Design review of the part built by this model. Coordinates are the model's own, in mm. A direction names the side the tool comes from. Coordinates: 2 decimals unless noted, no trailing zeros. Loops run counter-clockwise (first coordinate to the right, second up) from the corner with the lowest first, then second, coordinate; pieces in that order, holes last. Notation, with made-up numbers: (87, -32) - (120, -32) arc R23 cw to (120, -22) - close; hole circle Ø4 at (59, 80.25). An arc over 180 degrees is marked (long way). Return JSON: item names as keys, results as strings. Group by question number.
from build123d import *

# Parameters (mm, degrees)
BOSS_EXTRUDE1_DEPTH = 5.588
CUT_EXTRUDE1_REACH  = 80.367
SKETCH2_W           = 75.3618
SKETCH2_H           = 1.524
SKETCH3_W           = 8.255
SKETCH3_H           = 10.8204
CUT_EXTRUDE2_DEPTH  = 83.86461998


with BuildPart() as part:
    # Sketch1 → Boss-Extrude1 (new, symmetric)
    with BuildSketch(Plane.XY):
        Polygon((37.6809, 28.1432), (-37.6809, 28.1432), (-37.6809, 34.109215507), (-52.6415, 34.109215507), (-52.6415, 21.028215507), (-29.263085056, 21.028215507), (-18.341239915, -12.742623419), (-18.341239915, -29.6418), (-10.721239915, -29.6418), (-2.406356809, -15.24), (2.406356809, -15.24), (10.721239915, -29.6418), (18.341239915, -29.6418), (18.341239915, -12.742623419), (29.263085056, 21.028215507), (52.6415, 21.028215507), (52.6415, 34.109215507), (37.6809, 34.109215507), align=None)
        with BuildLine():
            Line((11.480303153, -7.62), (-11.480303153, -7.62))
            ThreePointArc((-11.480303153, -7.62), (-13.362052491, -6.011722817), (-12.066505741, -3.902435097))
            Line((-12.066505741, -3.902435097), (0, 0))
            Line((0, 0), (12.066505741, -3.902435097))
            ThreePointArc((12.066505741, -3.902435097), (13.362052491, -6.011722817), (11.480303153, -7.62))
        make_face(mode=Mode.SUBTRACT)
        Polygon((20.32, 22.225), (-20.32, 22.225), (0, 7.62), align=None, mode=Mode.SUBTRACT)
        Polygon((-21.301071122, 15.641859193), (-5.650084624, 4.392712647), (-16.52547404, 0.87549712), align=None, mode=Mode.SUBTRACT)
        Polygon((16.52547404, 0.87549712), (21.301071122, 15.641859193), (5.650084624, 4.392712647), align=None, mode=Mode.SUBTRACT)
    extrude(amount=BOSS_EXTRUDE1_DEPTH, both=True)

    # Cut-Extrude1: up to this face of the body (flat: up to its plane)
    cut_extrude1_end = Plane(part.part.faces().sort_by_distance((-14.531239915, -29.6418, 0))[0])
    # Sketch2 → Cut-Extrude1 (cut, up to the picked face)
    with BuildSketch(Plane(origin=(0, 28.1432, 0), x_dir=(1, 0, 0), z_dir=(0, 1, 0)), mode=Mode.PRIVATE) as cut_extrude1_sk1:
        with Locations((0, -4.826)):
            Rectangle(SKETCH2_W, SKETCH2_H)
    cut_extrude1_tool1 = split(extrude(cut_extrude1_sk1.sketch, amount=-CUT_EXTRUDE1_REACH, mode=Mode.PRIVATE), bisect_by=cut_extrude1_end, keep=Keep.BOTH, mode=Mode.PRIVATE)
    # Sketch2 → Cut-Extrude1 (cut, up to the picked face)
    with BuildSketch(Plane(origin=(0, 28.1432, 0), x_dir=(1, 0, 0), z_dir=(0, 1, 0)), mode=Mode.PRIVATE) as cut_extrude1_sk2:
        with Locations((0, 4.826)):
            Rectangle(SKETCH2_W, SKETCH2_H)
    cut_extrude1_tool2 = split(extrude(cut_extrude1_sk2.sketch, amount=-CUT_EXTRUDE1_REACH, mode=Mode.PRIVATE), bisect_by=cut_extrude1_end, keep=Keep.BOTH, mode=Mode.PRIVATE)
    add(cut_extrude1_tool1.solids().sort_by(Axis((0, 28.1432, 4.826), (0, -1, 0)))[0], mode=Mode.SUBTRACT)
    add(cut_extrude1_tool2.solids().sort_by(Axis((0, 28.1432, -4.826), (0, -1, 0)))[0], mode=Mode.SUBTRACT)

    # Sketch3 → Cut-Extrude2 (cut, through all)
    with BuildSketch(Plane(origin=(0, 34.109215507, 0), x_dir=(1, 0, 0), z_dir=(0, 1, 0))):
        with Locations((-45.593, 0)):
            Rectangle(SKETCH3_W, SKETCH3_H)
        with Locations((45.593, 0)):
            Rectangle(SKETCH3_W, SKETCH3_H)
    extrude(amount=-CUT_EXTRUDE2_DEPTH, mode=Mode.SUBTRACT)


solid = part.part
Item 1: For faces 4 (the face through (1, 28.143, 0)), 5 (the face through (0, -7.62, 0)), 6 (the face through (49.72, 28, 0)), list the 3-axis set-ups (+Z, -Z, +X, -X, +Y, -Y) from which the entire face can be reached by the end or side of a thin tool; tool diameter is ignored.
Item 2: For P1, Ø2.5, axis at y = -23.5, z = 0, coming from the +X side; P2, Ø5, axis at x = 24, z = -4.5, coming from the +Y side; P3, Ø4, axis at y = -21, z = -2, coming from the -X side, all flat-tipped, find the tip position at first contact; note any pin that passes through.
Item 3: To check wall thickness, follow line 1 (X direction, y = 23.5, z = 2.75); line 2 (X direction, y = 31, z = 0); line 3 (Y direction, x = 9.5, z = 3.5) (3 decimals). State the ranges of each line that lie inside material, in increasing order. Write a range as from..to.
Item 4: Draft analysis for pull direction Z (two halves, no side actions). For faces 1 (the face through (-1, 6, 4.064)), 2 (the face through (-41.466, 28, 0)), 3 (the face through (-39, 21.028, 0)), state which applies: pulls with the +Z half, pulls with the -Z half, needs draft (parallel to the pull), parting line crosses it, or undercut.
Item 5: Add section D-D (x = 40). State the section outline as (y, z) points, then the cut area to 3 significant figures.
Item 6: Add section A-A (z = -3). Give the number of separate pieces and of enclosed holes in the cut face, then the cut area to 3 significant figures.
Item 7: Add section C-C (y = 2). State the section outline as (x, z) points.
Item 8: Add section B-B (y = 17). State the section outline as (x, z) points, then the cut area to 3 significant figures.
Answers below:
{
 "1": {"face 4": "+Z, -Z, +Y", "face 5": "+Z, -Z", "face 6": "+Y, -Y"},
 "2": {"P1": "stops at x = 18.34", "P2": "stops at y = 28.14", "P3": "stops at x = -18.34"},
 "3": {"line 1": "x = -52.64..-49.72, -41.47..41.47, 49.72..52.64", "line 2": "x = -52.64..-49.72, -41.47..-37.68, 37.68..41.47, 49.72..52.64", "line 3": "y = -27.527..-7.62, -3.072..3.148, 7.16..14.448, 22.225..28.143"},
 "4": {"face 1": "pulls with the +Z half", "face 2": "undercut", "face 3": "needs draft"},
 "5": {"outline": "(21.03, -5.59) - (34.11, -5.59) - (34.11, 5.59) - (21.03, 5.59) - close", "area": "146 mm^2"},
 "6": {"separate pieces": "3", "enclosed holes": "4", "area": "2,130 mm^2"},
 "7": {"outline": "(-23.11, -4.06) - (-16.89, -4.06) - (-16.89, 4.06) - (-23.11, 4.06) - close; (-13.05, -4.06) - (13.05, -4.06) - (13.05, 4.06) - (-13.05, 4.06) - close; (16.89, -4.06) - (23.11, -4.06) - (23.11, 4.06) - (16.89, 4.06) - close"},
 "8": {"outline": "(-27.96, -4.06) - (-13.05, -4.06) - (-13.05, 4.06) - (-27.96, 4.06) - close; (13.05, -4.06) - (27.96, -4.06) - (27.96, 4.06) - (13.05, 4.06) - close", "area": "242 mm^2"}
}
